Can you work these out from the model? Positions are in its coordinate system, mm. A direction names the side the tool comes from. Give positions to 0.01 mm unless a question says otherwise; leave off trailing zeros. Loops run counter-clockwise (first coordinate to the right, second up) from the corner with the lowest first, then second, coordinate; pieces in that order, holes last. Notation, with made-up numbers: M 22.5,53.5 L 54.5,53.5 A32 ccw 54.5,87.5 Z; hole C -33.75,80.25 d6. An arc over 180 degrees is marked long. Answer as a JSON object with one key per item and string values.
```python
from build123d import *

# Parameters (mm, degrees)
SKETCH018_R           = 1.5
POCKET002_DEPTH       = 5
POLARPATTERN001_COUNT = 6
SKETCH019_W           = 44.124263
SKETCH019_H           = 42
POCKET003_DEPTH       = 27
SKETCH020_R           = 3
POCKET004_DEPTH       = 20
SKETCH021_W           = 55.928879
SKETCH021_H           = 10.367922
POCKET005_DEPTH       = 5


with BuildPart() as part:
    # Sketch017 → Revolution001 (revolve)
    with BuildSketch(Plane.XZ):
        Polygon((14, 0), (14, 5), (22, 5), (22, 32), (32.5, 32), (32.5, 5), (36.5, 5), (36.5, 0), align=None)
    revolve(axis=Axis((0, 0, 0), (0, 0, 1)))

    # Sketch018 (on Face2 of Revolution001) → Pocket002 (cut)
    with BuildSketch(Plane(origin=(0, 0, 5), x_dir=(-1, 0, 0), z_dir=(0, 0, 1))):
        with Locations((0, 19)):
            Circle(SKETCH018_R)
    pocket002 = extrude(amount=-POCKET002_DEPTH, mode=Mode.SUBTRACT)

    # PolarPattern001: Pocket002 ×6 about axis
    polarpattern001_axis = Axis((0, 0, 5), (0, 0, 1))
    for i in range(1, POLARPATTERN001_COUNT):
        add(pocket002.rotate(polarpattern001_axis, i * 360 / POLARPATTERN001_COUNT), mode=Mode.SUBTRACT)

    # Sketch019 (on Face13 of PolarPattern001) → Pocket003 (cut)
    with BuildSketch(Plane(origin=(0, 0, 32), x_dir=(-1, 0, 0), z_dir=(0, 0, 1))):
        with Locations((-25.154536, 0)):
            Rectangle(SKETCH019_W, SKETCH019_H)
    extrude(amount=-POCKET003_DEPTH, mode=Mode.SUBTRACT)

    # Sketch020 (on Face14 of Pocket003) → Pocket004 (cut)
    with BuildSketch(Plane(origin=(0, 0, 32), x_dir=(-1, 0, 0), z_dir=(0, 0, 1))):
        with Locations((0, 27)):
            Circle(SKETCH020_R)
        with Locations((0, -27)):
            Circle(SKETCH020_R)
        with Locations((27, 0)):
            Circle(SKETCH020_R)
    extrude(amount=-POCKET004_DEPTH, mode=Mode.SUBTRACT)

    # Sketch021 (on Face2 of Pocket004) → Pocket005 (cut)
    with BuildSketch(Plane(origin=(0, 0, 5), x_dir=(-1, 0, 0), z_dir=(0, 0, 1))):
        with Locations((-39.002113, 0)):
            Rectangle(SKETCH021_W, SKETCH021_H)
    extrude(amount=-POCKET005_DEPTH, mode=Mode.SUBTRACT)


with BuildPart() as part_1:
    # Body placement: moved
    add(part.part.moved(Location((0, -3e-06, 29.000002))))


solid = part_1.part
```
1) Suppose I cut it at C-C, the plane x = 11.5. Write out the boundary of the cut face in (y, z), and give its area (3 significant figures).
Answer list:
{"outline": "M -34.64,29 L -7.98,29 L -7.98,34 L -21,34 L -21,61 L -30.4,61 L -30.4,34 L -34.64,34 Z; M 7.98,29 L 34.64,29 L 34.64,34 L 30.4,34 L 30.4,61 L 21,61 L 21,34 L 7.98,34 Z", "area": "774 mm^2"}
2) Please list where these lines run through material, in increasing order: line 1 along Y through (x, z) = (0, 53); line 2 along Y through (x, z) = (0, 31.45); line 3 along Y through (x, z) = (-11, 55). Write a range as from..to.
Answer list:
{"line 1": "-32.5..-30, -24..-22, 22..24, 30..32.5", "line 2": "-36.5..-20.5, -17.5..-14, 14..17.5, 20.5..36.5", "line 3": "-30.58..-19.05, 19.05..30.58"}
3) Suppose I cut it at D-D, the plane y = 2. Write out the boundary of the cut face in (x, z).
Answer list:
{"outline": "M -36.45,29 L -13.86,29 L -13.86,34 L -21.91,34 L -21.91,61 L -24.76,61 L -24.76,41 L -29.24,41 L -29.24,61 L -32.44,61 L -32.44,34 L -36.45,34 Z"}
4) If we mould it in two halves opening along Y, with no side actions, what happens to faces 5 (the flat face through (0, 27, 41)), 6 (the flat face through (-23, 0, 61)), 7 (the cylindrical face through (-36.468, 1.532, 31.465))? For each: +Y half, -Y half, draft (parallel to the pull), parting line (faces both ways), or undercut.
Answer list:
{"face 5": "undercut", "face 6": "draft", "face 7": "parting line"}
5) Suppose I cut it at A-A, the plane x = 0. Give the number of separate pieces and of enclosed holes in the cut face, and give its area (3 significant figures).
Answer list:
{"separate pieces": "4", "enclosed holes": "0", "area": "522 mm^2"}
6) Will these pins go through, and if not, where does the flat tip stop? pin 1 Ø12 at (x, z) = (3.5, 44.5) entering from -Y; pin 2 Ø1.5 at (y, z) = (-21.5, 51.5) entering from -X; pin 3 Ø4 at (x, y) = (-16.45, -9.5) entering from +Z; pin 4 Ø1.8 at (x, y) = (16.45, -9.5) entering from -Z.
Answer list:
{"pin 1": "y = -32.5", "pin 2": "x = -25.01", "pin 3": "z = 34", "pin 4": "through"}
7) For faces 1 (the cylindrical face through (15.349, -8.486, 31.535)), 2 (the flat face through (16, -21, 48)), 3 (the cylindrical face through (-24, 0, 51)), 4 (the flat face through (25, 5.184, 32)), which set-ups out of +Z, -Z, +X, -X, +Y, -Y let a thin tool reach every point of the face, with its end or its side?
Answer list:
{"face 1": "+Z, -Z", "face 2": "+Z, +X", "face 3": "+Z", "face 4": "+Z, -Z, +X"}
8) Suppose I cut it at B-B, the plane z = 45.5. Write out the boundary of the cut face in (x, y), and give its area (3 significant figures).
Answer list:
{"outline": "M 6.56,-21 A22 cw long 6.56,21 L 24.8,21 A32.5 ccw long 24.8,-21 Z; hole C -27,0 d6; hole C 0,-27 d6; hole C 0,27 d6", "area": "1,200 mm^2"}
